Source: CAD feature listing. Evaluate the final solid. Frame: model axes, mm. Give positions to 0.01 mm unless a question says otherwise; leave off trailing zeros. Write each loop counter-clockwise with the first axis right and the second up, starting at its lowest first coordinate (ties: lowest second). Pieces come first, ordered by that corner, then holes. Notation, with made-up numbers: (-36.5, 1) -> (-7.5, 1) arc R10 ccw to (-7.5, 8) -> close; hole circle Ø2 at (-9.75, 44.5). An arc over 180 degrees is marked (long way). Use one line per item in the form item = value. Start each with the question number.
(1) First-contact query: P1, Ø1, axis at x = -1.5, z = 0.5, coming from the +Y side. Flat tip, straight axial feed; report the tip coordinate or a pass-through.
(2) Cut plane B-B, the plane z = 0. Count the separate pieces of the cut face and the enclosed holes in it, and give its area (3 significant figures).
(3) Material intervals for line 1 along X through (y, z) = (3.4, -0.05); line 2 along Z through (x, y) = (-0.85, 3.7); line 3 along Z through (x, y) = (1.8, 1.3), sorted ascending. Write a range as from..to.
(4) Draft query along X for faces 1 (the face through (-0.23, 0.51, 2.12)), 2 (the face through (-0.434, 3.493, 1.952)). Return one class per face: pulls with the +X half, pulls with the -X half, needs draft (parallel to the pull), parting line crosses it, or undercut.
(5) Cut plane C-C, the plane y = 1.35. Output: boundary loops of the cut face in (x, z), and give its area (3 significant figures).
from build123d import *

# Parameters (mm, degrees)
SKETCH1_R           = 2
SKETCH1_R_2         = 1.5
BOSS_EXTRUDE1_DEPTH = 4
CUT_EXTRUDE3_DEPTH  = 5
CHAMFER1_SIZE       = 0.25


with BuildPart() as part:
    # Sketch1 → Boss-Extrude1 (new body)
    with BuildSketch(Plane(origin=(0, 0, 0), x_dir=(1, 0, 0), z_dir=(0, 1, 0))):
        Circle(SKETCH1_R)
        Circle(SKETCH1_R_2, mode=Mode.SUBTRACT)
    extrude(amount=BOSS_EXTRUDE1_DEPTH)

    # Sketch2 → Revolve1 (revolve)
    with BuildSketch(Plane.XY):
        Polygon((2, 3), (2.5, 2.711324865), (2.5, 1.788675135), (2, 1.5), align=None)
        Polygon((2, 0), (2.5, 0), (2.5, 0.711324865), (2, 1), align=None)
    revolve(axis=Axis((0, 0, 0), (0, 1, 0)))

    # Sketch3 → Cut-Extrude3 (cut, through all)
    with BuildSketch(Plane(origin=(0, 4, 0), x_dir=(1, 0, 0), z_dir=(0, 1, 0))):
        with BuildLine():
            Line((-0.883481791, 1.794285352), (0.462232224, 2.456896695))
            ThreePointArc((0.462232224, 2.456896695), (-0.058686206, 2.499311091), (-0.577039766, 2.432493599))
            Line((-0.577039766, 2.432493599), (-0.883481791, 1.794285352))
        make_face()
        with BuildLine():
            Line((0.462232224, 2.456896695), (-0.077299176, 1.998505651))
            Line((-0.077299176, 1.998505651), (1.421580063, 2.056480033))
            ThreePointArc((1.421580063, 2.056480033), (0.962948887, 2.307104125), (0.462232224, 2.456896695))
        make_face()
        with BuildLine():
            ThreePointArc((2.135123794, 1.30047929), (1.818081368, 1.715977896), (1.421580063, 2.056480033))
            Line((1.421580063, 2.056480033), (0.742249169, 1.857166167))
            Line((0.742249169, 1.857166167), (2.135123794, 1.30047929))
        make_face()
        with BuildLine():
            ThreePointArc((2.479485224, 0.319613864), (2.358851064, 0.8281435), (2.135123794, 1.30047929))
            Line((2.135123794, 1.30047929), (1.433455889, 1.394705781))
            Line((1.433455889, 1.394705781), (2.479485224, 0.319613864))
        make_face()
        with BuildLine():
            ThreePointArc((2.5, 0), (2.494866035, 0.160135785), (2.479485224, 0.319613864))
            Line((2.479485224, 0.319613864), (1.876805063, 0.691088094))
            Line((1.876805063, 0.691088094), (2.395121134, -0.716515703))
            ThreePointArc((2.395121134, -0.716515703), (2.473641328, -0.362075382), (2.5, 0))
        make_face()
        with BuildLine():
            ThreePointArc((1.896618841, -1.628753196), (2.193809999, -1.198831801), (2.395121134, -0.716515703))
            Line((2.395121134, -0.716515703), (1.995637592, -0.132025002))
            Line((1.995637592, -0.132025002), (1.896618841, -1.628753196))
        make_face()
        with BuildLine():
            ThreePointArc((1.07017392, -2.259364464), (1.516536338, -1.987490261), (1.896618841, -1.628753196))
            Line((1.896618841, -1.628753196), (1.769406251, -0.932309776))
            Line((1.769406251, -0.932309776), (1.07017392, -2.259364464))
        make_face()
        with BuildLine():
            ThreePointArc((0.058686206, -2.499311091), (0.577039766, -2.432493599), (1.07017392, -2.259364464))
            Line((1.07017392, -2.259364464), (1.237228495, -1.57138972))
            Line((1.237228495, -1.57138972), (0.058686206, -2.499311091))
        make_face()
        with BuildLine():
            ThreePointArc((-0.962948887, -2.307104125), (-0.462232224, -2.456896695), (0.058686206, -2.499311091))
            Line((0.058686206, -2.499311091), (0.491122692, -1.938762105))
            Line((0.491122692, -1.938762105), (-0.962948887, -2.307104125))
        make_face()
        with BuildLine():
            Line((-0.339902686, -1.97090491), (-1.818081368, -1.715977896))
            ThreePointArc((-1.818081368, -1.715977896), (-1.421580063, -2.056480033), (-0.962948887, -2.307104125))
            Line((-0.962948887, -2.307104125), (-0.339902686, -1.97090491))
        make_face()
        with BuildLine():
            Line((-1.112155801, -1.662260351), (-2.358851064, -0.8281435))
            ThreePointArc((-2.358851064, -0.8281435), (-2.135123794, -1.30047929), (-1.818081368, -1.715977896))
            Line((-1.818081368, -1.715977896), (-1.112155801, -1.662260351))
        make_face()
        with BuildLine():
            Line((-1.692107076, -1.066195875), (-2.491753982, 0.202884431))
            ThreePointArc((-2.491753982, 0.202884431), (-2.479485224, -0.319613864), (-2.358851064, -0.8281435))
            Line((-2.358851064, -0.8281435), (-1.692107076, -1.066195875))
        make_face()
        with BuildLine():
            Line((-1.979477664, -0.285776447), (-2.193809999, 1.198831801))
            ThreePointArc((-2.193809999, 1.198831801), (-2.395121134, 0.716515703), (-2.491753982, 0.202884431))
            Line((-2.491753982, 0.202884431), (-1.979477664, -0.285776447))
        make_face()
        with BuildLine():
            Line((-1.924578581, 0.544056325), (-1.516536338, 1.987490261))
            ThreePointArc((-1.516536338, 1.987490261), (-1.896618841, 1.628753196), (-2.193809999, 1.198831801))
            Line((-2.193809999, 1.198831801), (-1.924578581, 0.544056325))
        make_face()
        with BuildLine():
            Line((-1.536902378, 1.279816816), (-0.577039766, 2.432493599))
            ThreePointArc((-0.577039766, 2.432493599), (-1.07017392, 2.259364464), (-1.516536338, 1.987490261))
            Line((-1.516536338, 1.987490261), (-1.536902378, 1.279816816))
        make_face()
    extrude(amount=-CUT_EXTRUDE3_DEPTH, mode=Mode.SUBTRACT)

    # Chamfer1
    chamfer1_edges = [part.edges().sort_by_distance(p)[0] for p in [
        (-1.5, 0, 0),
        (-1.5, 4, 0),
    ]]
    chamfer(chamfer1_edges, length=CHAMFER1_SIZE)


solid = part.part
Geometry says:
q1.P1 = 4
q2.separate_pieces = 4
q2.enclosed_holes = 0
q2.area = 4.40 mm^2
q3.line_1 = -2..-1.5, 1.5..2
q3.line_2 = -1.81..-1.24, 1.24..1.81
q3.line_3 = -0.87..0.87
q4.face_1 = undercut
q4.face_2 = parting line crosses it
q5.outline = circle Ø4 at (0, 0); hole circle Ø3 at (0, 0)
q5.area = 5.50 mm^2
